from build123d import *

# Parameters (mm, degrees)
CROQUIS1_R                 = 2.1
SALIENTE_EXTRUIR1_DEPTH    = 2
CROQUIS4_W                 = 49
CROQUIS4_H                 = 23
SALIENTE_EXTRUIR3_DEPTH    = 2
SALIENTE_EXTRUIR4_DEPTH    = 24
CROQUIS7_W                 = 10
CROQUIS7_H                 = 16
CROQUIS7_W_2               = 41
SALIENTE_EXTRUIR5_DEPTH    = 2
CROQUIS8_R                 = 2.1
SALIENTE_EXTRUIR6_DEPTH    = 2
CROQUIS9_W                 = 41
CROQUIS9_H                 = 2
CROQUIS9_W_2               = 10
SALIENTE_EXTRUIR7_DEPTH    = 12
SALIENTE_EXTRUIR8_REACH    = 99.227
SALIENTE_EXTRUIR9_DEPTH    = 2
SALIENTE_EXTRUIR10_DEPTH   = 2
CROQUIS15_W                = 80
CROQUIS15_H                = 8.5
SALIENTE_EXTRUIR11_DEPTH   = 2
CROQUIS16_W                = 48
CROQUIS16_H                = 14
SALIENTE_EXTRUIR12_DEPTH   = 2
SALIENTE_EXTRUIR13_DEPTH   = 16.5
CORTAR_EXTRUIR1_DEPTH      = 116.347301659
CORTAR_EXTRUIR1_DEPTH_BACK = 6


with BuildPart() as part:
    # Croquis1 → Saliente-Extruir1 (new body)
    with BuildSketch(Plane(origin=(0, 0, 0), x_dir=(1, 0, 0), z_dir=(0, 1, 0))):
        Polygon((50, 8), (50, -41), (9, -41), (9, -6), (-40, -6), (-40, -41), (-50, -41), (-50, 8), align=None)
        with Locations(Location((46, 0, 0), (0, 0, 270))):
            Circle(CROQUIS1_R, mode=Mode.SUBTRACT)
        with Locations(Location((-46, 0, 0), (0, 0, 270))):
            Circle(CROQUIS1_R, mode=Mode.SUBTRACT)
    extrude(amount=SALIENTE_EXTRUIR1_DEPTH)



with BuildPart() as body_2:
    # Croquis4 → Saliente-Extruir3 (new body)
    with BuildSketch(Plane(origin=(0, 12, 0), x_dir=(1, 0, 0), z_dir=(0, 1, 0))):
        with Locations((-15.5, -64.5)):
            Rectangle(CROQUIS4_W, CROQUIS4_H)
    extrude(amount=-SALIENTE_EXTRUIR3_DEPTH)

    # Croquis6 → Saliente-Extruir4 (add)
    with BuildSketch(Plane.XZ.offset(-10)):
        Polygon((-38, 74), (7, 74), (7, 53), (9, 53), (9, 76), (-40, 76), (-40, 53), (-38, 53), align=None)
    extrude(amount=SALIENTE_EXTRUIR4_DEPTH)

    # Croquis7 → Saliente-Extruir5 (add)
    with BuildSketch(Plane.XY.offset(53)):
        with Locations((-45, -6)):
            Rectangle(CROQUIS7_W, CROQUIS7_H)
        with Locations((29.5, -6)):
            Rectangle(CROQUIS7_W_2, CROQUIS7_H)
    extrude(amount=SALIENTE_EXTRUIR5_DEPTH)

    # Croquis8 → Saliente-Extruir6 (add)
    # profile 1 of 2: a face of its own
    with BuildSketch(Plane.XZ.offset(14)):
        with BuildLine():
            Line((30, 55), (50, 55))
            Line((50, 55), (50, 62))
            ThreePointArc((50, 62), (47.788854382, 65.577708764), (43.6, 65.2))
            Line((43.6, 65.2), (30, 55))
        make_face()
        with Locations(Location((46, 62, 0), (0, 0, 270))):
            Circle(CROQUIS8_R, mode=Mode.SUBTRACT)
    # profile 2 of 2: a face of its own
    with BuildSketch(Plane.XZ.offset(14)):
        with BuildLine():
            Line((-40, 55), (-40, 76))
            Line((-40, 76), (-49.133743765, 64.485890185))
            ThreePointArc((-49.133743765, 64.485890185), (-49.777232787, 63.316249395), (-50, 62))
            Line((-50, 62), (-50, 55))
            Line((-50, 55), (-40, 55))
        make_face()
        with Locations(Location((-46, 62, 0), (0, 0, 270))):
            Circle(CROQUIS8_R, mode=Mode.SUBTRACT)
    extrude(amount=-SALIENTE_EXTRUIR6_DEPTH)


with BuildPart() as part_1:
    add(part.part)

    add(body_2.part)  # Saliente-Extruir7 merges body 2
    # Croquis9 → Saliente-Extruir7 (add)
    with BuildSketch(Plane.XY.offset(41)):
        with Locations((29.5, 1)):
            Rectangle(CROQUIS9_W, CROQUIS9_H)
        with Locations((-45, 1)):
            Rectangle(CROQUIS9_W_2, CROQUIS9_H)
    extrude(amount=SALIENTE_EXTRUIR7_DEPTH)

    # Saliente-Extruir8: up to this face of the body (flat: up to its plane)
    saliente_extruir8_end = Plane(part_1.part.faces().sort_by_distance((-40, 0.267175573, 65.061068702))[0])
    # Croquis12 → Saliente-Extruir8 (add, up to the picked face)
    with BuildSketch(Plane.ZY.offset(-9), mode=Mode.PRIVATE) as saliente_extruir8_sk1:
        Polygon((53, 10), (53, 12), (6, 2), (6, 0), align=None)
    saliente_extruir8_tool1 = split(extrude(saliente_extruir8_sk1.sketch, amount=SALIENTE_EXTRUIR8_REACH, mode=Mode.PRIVATE), bisect_by=saliente_extruir8_end, keep=Keep.BOTH, mode=Mode.PRIVATE)
    add(saliente_extruir8_tool1.solids().sort_by(Axis((9, 6, 29.5), (-1, 0, 0)))[0])

    # Croquis13 → Saliente-Extruir9 (add)
    with BuildSketch(Plane(origin=(9, 0, 0), x_dir=(0, 0, -1), z_dir=(1, 0, 0))):
        Polygon((-53, 12), (-53, 0), (-6, 0), (-6, 2), align=None)
    extrude(amount=-SALIENTE_EXTRUIR9_DEPTH)

    # Croquis14 → Saliente-Extruir10 (add)
    with BuildSketch(Plane(origin=(-40, 0, 0), x_dir=(0, 0, -1), z_dir=(1, 0, 0))):
        Polygon((-6, 0), (-6, 2), (-53, 10), (-53, 0), align=None)
    extrude(amount=SALIENTE_EXTRUIR10_DEPTH)

    # Croquis15 → Saliente-Extruir11 (add)
    with BuildSketch(Plane(origin=(0, 0, -8), x_dir=(-1, 0, 0), z_dir=(0, 0, -1))):
        with Locations((0, -2.25)):
            Rectangle(CROQUIS15_W, CROQUIS15_H)
    extrude(amount=-SALIENTE_EXTRUIR11_DEPTH)

    # Croquis16 → Saliente-Extruir12 (add)
    with BuildSketch(Plane.XZ.offset(6.5)):
        Polygon((40, -6), (40, -13), (26, -13), (26, -27), (-26, -27), (-26, -13), (-40, -13), (-40, -6), align=None)
        with Locations((0, -18)):
            Rectangle(CROQUIS16_W, CROQUIS16_H, mode=Mode.SUBTRACT)
    extrude(amount=-SALIENTE_EXTRUIR12_DEPTH)

    # Croquis17 → Saliente-Extruir13 (add)
    with BuildSketch(Plane(origin=(0, -4.5, 0), x_dir=(1, 0, 0), z_dir=(0, 1, 0))):
        Polygon((-24, 25), (24, 25), (24, 11), (38.139050544, 11), (40, 11), (40, 13), (26, 13), (26, 27), (-26, 27), (-26, 13), (-40, 13), (-40, 11), (-38.139050544, 11), (-24, 11), align=None)
    extrude(amount=SALIENTE_EXTRUIR13_DEPTH)

    # Croquis18 → Cortar-Extruir1 (cut, two sides: drawn at the far end of the back side and taken through both)
    with BuildSketch(Plane(origin=(0, 0, -27), x_dir=(-1, 0, 0), z_dir=(0, 0, -1)).offset(-CORTAR_EXTRUIR1_DEPTH_BACK)):
        Polygon((-10, 152.782261794), (-10, 12), (-10, 9.75), (10, 9.75), (10, 12), (10, 152.782261794), (10, 434.346785383), (-10, 434.346785383), align=None)
    extrude(amount=CORTAR_EXTRUIR1_DEPTH + CORTAR_EXTRUIR1_DEPTH_BACK, mode=Mode.SUBTRACT)


solid = part_1.part
Model file for the job. Use its own axes, mm. A direction names the side the tool comes from. Give positions to 0.01 mm unless a question says otherwise; leave off trailing zeros. Loops run counter-clockwise (first coordinate to the right, second up) from the corner with the lowest first, then second, coordinate; pieces in that order, holes last. Notation, with made-up numbers: (79, -3) -> (101, -3) arc R21 cw to (101, 7) -> close; hole circle Ø1 at (-39, 6). An arc over 180 degrees is marked (long way). Use a Markdown table: item, result. Add a question column.
(1) Mould opens along Z. For faces 5 (the flat face through (32, 4, -11)), 6 (the flat face through (33, 3, -13)), 7 (the flat face through (-44.503, -13.014, 70.324)) say: +Z half, -Z half, draft (parallel to the pull), parting line (faces both ways), or undercut.
(2) Wall check: line 1 along X through (y, z) = (0.9, 0); line 2 along Z through (x, y) = (-6.5, -2.5); line 3 along X through (y, z) = (0, -17). Give the ranges that are in metal, low to high.
(3) Slice it at B-B on x = 46. List the corners of the cut face in (y, z).
(4) Slice it at D-D on z = 0. List the corners of the cut face in (x, y).
(5) Slice it at C-C on y = 5.75. List the corners of the cut face in (x, z) (3 decimals).
(6) Slice it at A-A on x = 20. List the corners of the cut face in (y, z).
(7) Tool access for faces 1 (the flat face through (1, -3, -6)), 2 (the flat face through (-32, 4, -11)), 3 (the flat face through (-16, -2, 74)), 4 (the flat face through (36.895, -13.014, 60.171)): list every direction of +Z, -Z, +X, -X, +Y, -Y with a clear straight run to the whole face (end or side of a thin tool).
(8) Drop flat-ended pins along their axis: pin 1 Ø2 at (x, y) = (37.5, 7.5) entering from -Z; pin 2 Ø1 at (y, z) = (5.5, 42) entering from -X; pin 3 Ø1 at (y, z) = (5, 40.5) entering from +X; pin 4 Ø4 at (x, z) = (-46, 0) entering from +Y. Give the stop position or say it passes through.
Filled sheet:
| question | item | result |
|---|---|---|
| 1 | face 5 | undercut |
| 1 | face 6 | -Z half |
| 1 | face 7 | +Z half |
| 2 | line 1 | -50 to -48.1, -43.9 to 43.9, 48.1 to 50 |
| 2 | line 2 | -27 to -25, -8 to -6, 74 to 76 |
| 2 | line 3 | -26 to -24, 24 to 26 |
| 3 | outline | (-14, 53) -> (0, 53) -> (0, 2.1) -> (2, 2.1) -> (2, 55) -> (-12, 55) -> (-12, 59.9) -> (-14, 59.9) -> close; (-14, 64.1) -> (-12, 64.1) -> (-12, 66) -> (-14, 66) -> close; (0, -8) -> (2, -8) -> (2, -2.1) -> (0, -2.1) -> close |
| 4 | outline | (-50, 0) -> (-48.1, 0) -> (-48.1, 2) -> (-50, 2) -> close; (-43.9, 0) -> (43.9, 0) -> (43.9, 2) -> (-43.9, 2) -> close; (48.1, 0) -> (50, 0) -> (50, 2) -> (48.1, 2) -> close |
| 5 | outline | (-40, -13) -> (-26, -13) -> (-26, -27) -> (26, -27) -> (26, -13) -> (40, -13) -> (40, -11) -> (24, -11) -> (24, -25) -> (-24, -25) -> (-24, -11) -> (-40, -11) -> close; (-40, 23.625) -> (9, 23.625) -> (9, 76) -> (-40, 76) -> close; hole (-38, 33.025) -> (7, 33.025) -> (7, 74) -> (-38, 74) -> close |
| 6 | outline | (-14, 53) -> (0, 53) -> (0, -6) -> (-6.5, -6) -> (-6.5, -11) -> (-4.5, -11) -> (-4.5, -8) -> (2, -8) -> (2, 55) -> (-14, 55) -> close; (-6.5, -27) -> (12, -27) -> (12, -25) -> (-6.5, -25) -> close |
| 7 | face 1 | +X, -X, -Y |
| 7 | face 2 | +X, -X, +Y |
| 7 | face 3 | -Y |
| 7 | face 4 | +Z, +Y, -Y |
| 8 | pin 1 | z = -13 |
| 8 | pin 2 | x = -40 |
| 8 | pin 3 | x = 9 |
| 8 | pin 4 | through |
